Autodesk Inventor part; units mm, degrees
ref_plane "YZ Plane" through (0, 0, 0) normal (1, 0, 0) x (0, 1, 0)
ref_plane "XZ Plane" through (0, 0, 0) normal (0, 1, 0) x (-1, 0, 0)
ref_plane "XY Plane" through (0, 0, 0) normal (0, 0, 1) x (1, 0, 0)
sketch "Sketch1" plane through (0, 0, 0) normal (0, 0, 1) x (1, 0, 0)
  line L0 (0, -22.0606) -> (0, 6.3638)
  line L1 (0, 2.2) -> (2.25, 2.2)
  line L2 (3.8, 0) -> (3.8, 0.56)
  arc A0 (3.8, 0.56) -> (2.25, 2.2) centre (0, -1.479) ccw
  line L3 (3.8, 0) -> (2, 0)
  line L4 (2, 0) -> (2, -10)
  line L5 (2, -10) -> (0, -10)
  point P0 (0, 0)
  dimension "BoltDia" = 4
  dimension "HeadDia" = 7.6
  dimension "HeadHeight" = 2.2
  dimension "SideHeight" = 0.56
  dimension "TopFlatDia" = 4.5
  dimension "Length" = 10
revolve "Revolution1" add sketch "Sketch1" angle 360 about axis through (0, -10, 0) along (0, 1, 0)
sketch "Sketch2" plane through (0, 2.2, 0) normal (0, 1, 0) x (1, 0, 0)
  circle A0 centre (0, 0) radius 2.25
  circle A1 centre (0, 0) radius 1.25 construction
  line L0 (-0.7217, 1.25) -> (0.7217, 1.25)
  line L1 (0.7217, 1.25) -> (1.4434, 0)
  line L2 (1.4434, 0) -> (0.7217, -1.25)
  line L3 (0.7217, -1.25) -> (-0.7217, -1.25)
  line L4 (-0.7217, -1.25) -> (-1.4434, 0)
  line L5 (-1.4434, 0) -> (-0.7217, 1.25)
  dimension "HexSize" = 2.5
extrude "Hex" cut sketch "Sketch2" against normal blind 1.3 contours L0 L1 L2 L3 L4 L5
thread "Thread1"
chamfer "Chamfer1" distance 0.4 angle 45 1 edges at (-2, -10, 0)
equation "\"d11\" = 0.1 * BoltDia"
equation "\"d12\" = 0.1 * BoltDia"
equation "\"d17\" = HexSize"
properties part number "SCREW, BUTTON HD, P, 12.9, M4X0.7X18MM" material "Steel"
Verification items for the finished model (mm, model axes). A direction names the side the tool comes from. Coordinates: 2 decimals unless noted, no trailing zeros. Order: outer loops, then holes, each group sorted by start corner. A loop starts at its lowest first (then second) coordinate and runs counter-clockwise, first axis right, second up. Notation, with made-up numbers: (35.25, 26) -> (75.25, 26) arc R23 cw to (75.25, 38) -> close; hole circle Ø3 at (65.5, -29). An arc over 180 degrees is marked (long way). Answer as CSV lines item,"result". Start each with the question number.
1) Set-up check for faces 4 (the face through (-1.08, 1.56, 0.63)), 5 (the face through (0, 2.2, 1.5)), 6 (the face through (2, 0, 2)): record each of +Z, -Z, +X, -X, +Y, -Y from which the full face is reachable in a straight line by a thin tool's end or side.
2) Release check for a two-part mould opening along X. For faces 1 (the face through (-1.088, 1.559, -0.616)), 2 (the face through (-3.796, 0.284, -0.167)), 3 (the face through (0, -10, 0)) record: released by +X, released by -X, zero draft, split by the parting line, or undercut.
3) Cross-section at A-A, the plane y = -6. Record the boundary of the cut face in (x, z).
4) Material ranges on L1, parallel to X at y = -2.25, z = 0; L2, parallel to Z at x = 0.5, y = 1; L3, parallel to X at y = -6, z = -1.5, recorded low to high. Write a range as [from, to].
5) Gauge pin test, flat ends, axial feed: pin 1 Ø1.5 at (y, z) = (0, 2.5) entering from -X; pin 2 Ø2 at (x, z) = (-0.5, 0) entering from +Y; pin 3 Ø3 at (y, z) = (-2, 2) entering from -X; pin 4 Ø1 at (x, y) = (0.5, 2) entering from +Z. Record the tip position at first contact, or that the pin passes through.
Conclusion:
1,face 4,"+Y"
1,face 5,"+Z, -Z, +X, -X, +Y"
1,face 6,"-Y"
2,face 1,"undercut"
2,face 2,"split by the parting line"
2,face 3,"zero draft"
3,outline,"circle Ø4 at (0, 0)"
4,L1,"x = [-2, 2]"
4,L2,"z = [-3.49, -1.25], [1.25, 3.49]"
4,L3,"x = [-1.32, 1.32]"
5,pin 1,"stops at x = -3.37"
5,pin 2,"stops at y = 2.2"
5,pin 3,"stops at x = -1.94"
5,pin 4,"stops at z = 3.08"
